Source: CAD feature listing. Evaluate the final solid. Frame: model axes, mm. Face numbers are marked on the shaded views. A direction names the side the tool comes from. Give positions to 0.01 mm unless a question says otherwise; leave off trailing zeros. Loops run counter-clockwise (first coordinate to the right, second up) from the corner with the lowest first, then second, coordinate; pieces in that order, holes last.
```python
from build123d import *

# Parameters (mm, degrees)
F0_R     = 7
F1_DEPTH = 5
F2_DEPTH = 3


with BuildPart() as f1:
    # F0 (on Top) → F1 (new body)
    with BuildSketch(Plane.XY):
        Circle(F0_R)
        with BuildLine():
            ThreePointArc((-1.75, -4.9497474683), (-5.25, 0), (-1.75, 4.9497474683))
            ThreePointArc((-1.75, 4.9497474683), (3.0310889132, 4.2866070499), (5.25, 0))
            ThreePointArc((5.25, 0), (3.0310889132, -4.2866070499), (-1.75, -4.9497474683))
        make_face(mode=Mode.SUBTRACT)
        with BuildLine():
            ThreePointArc((-1.75, -3.3166247904), (-3.75, 0), (-1.75, 3.3166247904))
            Line((-1.75, 3.3166247904), (-1.75, 4.9497474683))
            ThreePointArc((-1.75, 4.9497474683), (-5.25, 0), (-1.75, -4.9497474683))
            Line((-1.75, -4.9497474683), (-1.75, -3.3166247904))
        make_face()
        with BuildLine():
            Line((-1.75, 0), (-1.75, 3.3166247904))
            ThreePointArc((-1.75, 3.3166247904), (-3.75, 0), (-1.75, -3.3166247904))
            Line((-1.75, -3.3166247904), (-1.75, 0))
        make_face()
    extrude(amount=F1_DEPTH)

    # F0 (on Top) → F2 (join)
    with BuildSketch(Plane.XY):
        with BuildLine():
            ThreePointArc((-1.75, 3.3166247904), (1.9364916731, 3.2113081447), (3.75, 0))
            ThreePointArc((3.75, 0), (1.9364916731, -3.2113081447), (-1.75, -3.3166247904))
            Line((-1.75, -3.3166247904), (-1.75, -4.9497474683))
            ThreePointArc((-1.75, -4.9497474683), (3.0310889132, -4.2866070499), (5.25, 0))
            ThreePointArc((5.25, 0), (3.0310889132, 4.2866070499), (-1.75, 4.9497474683))
            Line((-1.75, 4.9497474683), (-1.75, 3.3166247904))
        make_face()
    extrude(amount=F2_DEPTH)


solid = f1.part
```
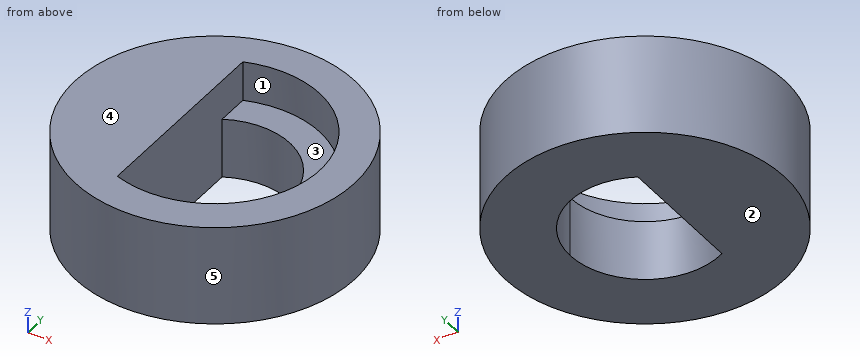
(1) First-contact query: pin 1 (2 mm diameter, centred on y = 3, z = 1, fed in from -X); pin 2 (1 mm diameter, centred on y = -5, z = 1, fed in from +X); pin 3 (1.5 mm diameter, centred on y = 2, z = 3, fed in from +X). Flat tips, straight axial feed; report the tip coordinate or a pass-through.
A:
pin 1: stops at x = -6.71
pin 2: stops at x = 5.36
pin 3: stops at x = 6.89
(2) Section D-D, the plane x = 1.5. Return the cut outline in (y, z), then the cut area to 3 significant figures.
A:
outline: (-6.84, 0) - (-3.44, 0) - (-3.44, 3) - (-5.03, 3) - (-5.03, 5) - (-6.84, 5) - close; (3.44, 0) - (6.84, 0) - (6.84, 5) - (5.03, 5) - (5.03, 3) - (3.44, 3) - close
area: 27.6 mm2
(3) Reachability of the marked faces 1 and 2 from +Z, -Z, +X, -X, +Y, -Y: full face, straight path, thin tool, end or side. Return the list, or none.
A:
face 1: +Z
face 2: -Z, +X, -X, +Y, -Y
(4) Section C-C, the plane z = 4.2. Return the cut outline in (x, y), then the cut area to 3 significant figures.
A:
outline: circle Ø14 at (0, 0); hole (-1.75, -4.95) arc R5.25 ccw (long way) to (-1.75, 4.95) - close
area: 92.6 mm2
(5) Section B-B, the plane y = 2.5. Return the cut outline in (x, z).
A:
outline: (-6.54, 0) - (-1.75, 0) - (-1.75, 5) - (-6.54, 5) - close; (2.8, 0) - (6.54, 0) - (6.54, 5) - (4.62, 5) - (4.62, 3) - (2.8, 3) - close
(6) Ray query, line 1 along Y through (x, z) = (0, 4.2); line 2 along Y through (x, z) = (2.5, 0.45); line 3 along X through (y, z) = (-0.5, 2.25). Return the intervals inside material, ascending.
A:
line 1: y = -7 to -5.25, 5.25 to 7
line 2: y = -6.54 to -2.8, 2.8 to 6.54
line 3: x = -6.98 to -1.75, 3.72 to 6.98
(7) Section A-A, the plane x = 0. Return the cut outline in (y, z), then the cut area to 3 significant figures.
A:
outline: (-7, 0) - (-3.75, 0) - (-3.75, 3) - (-5.25, 3) - (-5.25, 5) - (-7, 5) - close; (3.75, 0) - (7, 0) - (7, 5) - (5.25, 5) - (5.25, 3) - (3.75, 3) - close
area: 26.5 mm2
(8) Mould query, pull axis X, two halves, no side actions, for the marked faces 3, 4 and 5. Classes: pulls with the +X half, pulls with the -X half, needs draft (parallel to the pull), parting line crosses it, or undercut.
A:
face 3: undercut
face 4: needs draft
face 5: parting line crosses it
